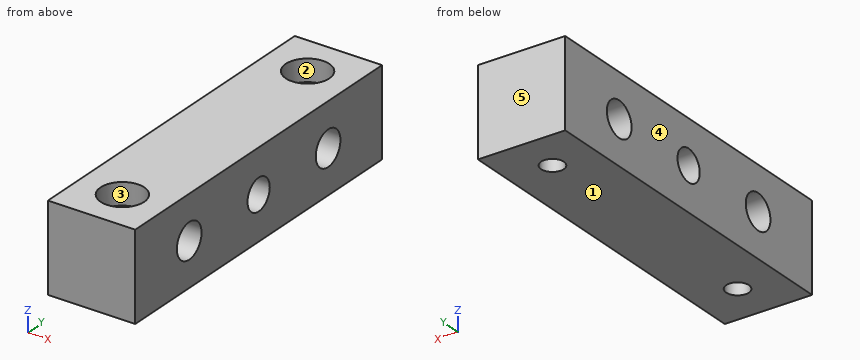
```python
from build123d import *

# Parameters (mm, degrees)
F0_W     = 20
F0_H     = 80
F0_R     = 2.6
F1_DEPTH = 20
F2_R     = 5
F3_DEPTH = 5
F4_R     = 4
F4_R_2   = 3.6
F5_DEPTH = 25


with BuildPart() as f1:
    # F0 (on Top) → F1 (new body)
    with BuildSketch(Plane.XY):
        Rectangle(F0_W, F0_H)
        with Locations((0, -30)):
            Circle(F0_R, mode=Mode.SUBTRACT)
        with Locations((0, 30)):
            Circle(F0_R, mode=Mode.SUBTRACT)
    extrude(amount=F1_DEPTH)

    # F2 (on face) → F3 (cut)
    with BuildSketch(Plane.XY.offset(20)):
        with Locations((0, 30)):
            Circle(F2_R)
        with Locations((0, -30)):
            Circle(F2_R)
    extrude(amount=-F3_DEPTH, mode=Mode.SUBTRACT)

    # F4 (on face) → F5 (cut)
    with BuildSketch(Plane.YZ.offset(10)):
        with Locations((-22.5, 10)):
            Circle(F4_R)
        with Locations((22.5, 10)):
            Circle(F4_R)
        with Locations((0, 10)):
            Circle(F4_R_2)
    extrude(amount=-F5_DEPTH, mode=Mode.SUBTRACT)


solid = f1.part
```
Here's how the part is built. I have some questions about the finished solid (model axes, mm). Face numbers are marked on the shaded views. A direction names the side the tool comes from. Coordinates: 2 decimals unless noted, no trailing zeros. Write each loop counter-clockwise with the first axis right and the second up, starting at its lowest first coordinate (ties: lowest second). Pieces come first, ordered by that corner, then holes. Notation, with made-up numbers: (35, -36) -> (91, -36) arc R10 ccw to (91, -23) -> close; hole circle Ø5 at (9.5, -1.5). An arc over 180 degrees is marked (long way). Use a Markdown table: item, result. Add a question column.
(1) If we section it at C-C, the plane z = 10: Write out the boundary of the cut face in (x, y), and give its area (3 significant figures).
(2) I'm going to push a flat-ended pin straight in: P1, Ø5, axis at x = 2, y = 30.5, coming from the +Z side. Where does the tip first touch, or does it pass through?
(3) If we section it at B-B, the plane y = 22.5: Write out the boundary of the cut face in (x, z), and give its area (3 significant figures).
(4) If we section it at D-D, the plane x = -4: Write out the boundary of the cut face in (y, z), and give its area (3 significant figures).
(5) We'd pull the mould along X, two halves only. Please class the marked faces 3, 4 and 5: +X half, -X half, draft (parallel to the pull), parting line (faces both ways), or undercut.
(6) Please list where these lines run through material, in increasing order: line 1 (Y direction, x = 0, z = 18.3); line 2 (Y direction, x = 0, z = 5.5); line 3 (Y direction, x = 6.25, z = 9.5).
(7) If we section it at A-A, the plane x = 0: Write out the boundary of the cut face in (y, z), and give its area (3 significant figures).
(8) For the marked faces 1 and 2, which set-ups out of +Z, -Z, +X, -X, +Y, -Y let a thin tool reach every point of the face, with its end or its side?
Outcome:
| question | item | result |
|---|---|---|
| 1 | outline | (-10, -40) -> (10, -40) -> (10, -26.5) -> (-10, -26.5) -> close; (-10, -18.5) -> (10, -18.5) -> (10, -3.6) -> (-10, -3.6) -> close; (-10, 3.6) -> (10, 3.6) -> (10, 18.5) -> (-10, 18.5) -> close; (-10, 26.5) -> (10, 26.5) -> (10, 40) -> (-10, 40) -> close; hole circle Ø5.2 at (0, -30); hole circle Ø5.2 at (0, 30) |
| 1 | area | 1,090 mm^2 |
| 2 | P1 | stops at z = 15 |
| 3 | outline | (-10, 0) -> (10, 0) -> (10, 6) -> (-10, 6) -> close; (-10, 14) -> (10, 14) -> (10, 20) -> (-10, 20) -> close |
| 3 | area | 240 mm^2 |
| 4 | outline | (-40, 0) -> (40, 0) -> (40, 20) -> (33, 20) -> (33, 15) -> (27, 15) -> (27, 20) -> (-27, 20) -> (-27, 15) -> (-33, 15) -> (-33, 20) -> (-40, 20) -> close; hole circle Ø8 at (-22.5, 10); hole circle Ø7.2 at (0, 10); hole circle Ø8 at (22.5, 10) |
| 4 | area | 1,400 mm^2 |
| 5 | face 3 | undercut |
| 5 | face 4 | -X half |
| 5 | face 5 | draft |
| 6 | line 1 | y = -40 to -35, -25 to 25, 35 to 40 |
| 6 | line 2 | y = -40 to -32.6, -27.4 to 27.4, 32.6 to 40 |
| 6 | line 3 | y = -40 to -26.47, -18.53 to -3.57, 3.57 to 18.53, 26.47 to 40 |
| 7 | outline | (-40, 0) -> (-32.6, 0) -> (-32.6, 15) -> (-35, 15) -> (-35, 20) -> (-40, 20) -> close; (-27.4, 0) -> (27.4, 0) -> (27.4, 15) -> (25, 15) -> (25, 20) -> (-25, 20) -> (-25, 15) -> (-27.4, 15) -> close; (32.6, 0) -> (40, 0) -> (40, 20) -> (35, 20) -> (35, 15) -> (32.6, 15) -> close; hole circle Ø8 at (-22.5, 10); hole circle Ø7.2 at (0, 10); hole circle Ø8 at (22.5, 10) |
| 7 | area | 1,200 mm^2 |
| 8 | face 1 | -Z, +X, -X, +Y, -Y |
| 8 | face 2 | +Z |
